The figure shows three views and two pictorial views of one solid part (mm, origin at its lowest corner). Answer the questions. A direction names the side the tool comes from. Coordinates: 2 decimals unless noted, no trailing zeros. Loops run counter-clockwise (first coordinate to the right, second up) from the corner with the lowest first, then second, coordinate; pieces in that order, holes last. Notation, with made-up numbers: (1, 1.25) - (12, 1.25) arc R34 ccw to (12, 32.25) - close; hole circle Ø5 at (-6, 56.25). An arc over 180 degrees is marked (long way). Return JSON: item names as keys, results as strings. Group by question number.
1. Section C-C (y = 31.5) is taken. Write down the section's boundary in (x, z), and give its area (3 significant figures).
2. The mould has two halves that part along X. Classify the marked faces 3 and 4: pulls with the +X half, pulls with the -X half, needs draft (parallel to the pull), parting line crosses it, or undercut.
3. Which of the six approach directions +Z, -Z, +X, -X, +Y, -Y give full straight-line access (tool end or side, diameter ignored) to the marked faces 1 and 2?
4. Section A-A (z = 31.75) is taken. Write down the section's boundary in (x, y) (3 decimals).
5. Find the intervals of material crossed by line 1 along Y through (x, z) = (59, 41) (3 decimals); line 2 along Y through (x, z) = (10, 31); line 3 along X through (y, z) = (13.5, 36), in increasing order.
6. Each of these flat-tipped pins is pushed along its axis until it touches: P1, Ø6, axis at y = 27.5, z = 26.5, coming from the -X side; P2, Ø1, axis at x = 52, z = 36.5, coming from the +Y side; P3, Ø6, axis at y = 22.5, z = 36.5, coming from the -X side. Where does it stop, or does it pass through?
7. Section B-B (x = 31.75) is taken. Write down the section's boundary in (y, z) (3 decimals), and give its area (3 significant figures).
8. Section D-D (x = 59.5) is taken. Write down the section's boundary in (y, z) (3 decimals).
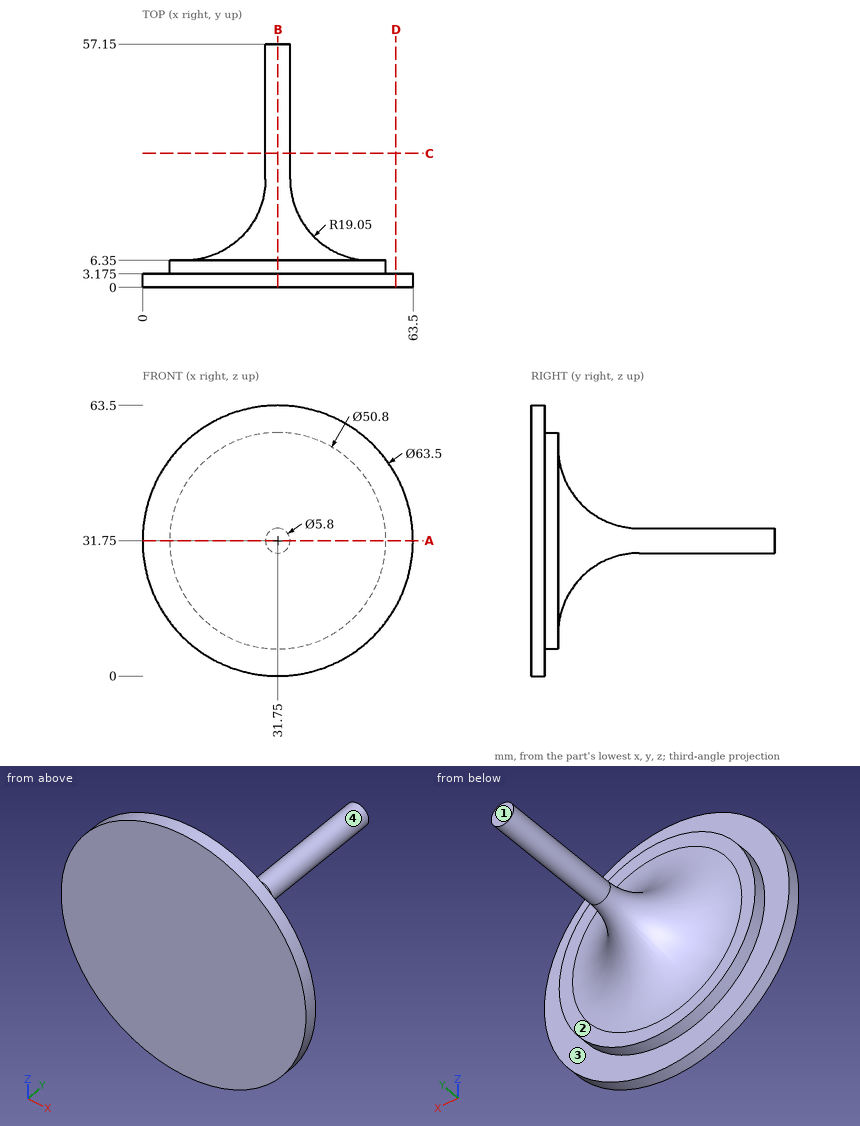
The answers:
{
 "1": {"outline": "circle Ø5.8 at (31.75, 31.75)", "area": "26.4 mm2"},
 "2": {"face 3": "needs draft", "face 4": "parting line crosses it"},
 "3": {"face 1": "+Z, -Z, +X, -X, +Y", "face 2": "+Y"},
 "4": {"outline": "(0, 0) - (63.5, 0) - (63.5, 3.175) - (57.15, 3.175) - (57.15, 6.35) - (53.7, 6.35) arc R19.05 cw to (34.65, 25.4) - (34.65, 57.15) - (28.85, 57.15) - (28.85, 25.4) arc R19.05 cw to (9.8, 6.35) - (6.35, 6.35) - (6.35, 3.175) - (0, 3.175) - close"},
 "5": {"line 1": "y = 0 to 3.175", "line 2": "y = 0 to 6.35", "line 3": "x = 26.09 to 37.41"},
 "6": {"P1": "stops at x = 29.92", "P2": "stops at y = 6.42", "P3": "stops at x = 29.06"},
 "7": {"outline": "(0, 0) - (3.175, 0) - (3.175, 6.35) - (6.35, 6.35) - (6.35, 9.8) arc R19.05 cw to (25.4, 28.85) - (57.15, 28.85) - (57.15, 34.65) - (25.4, 34.65) arc R19.05 cw to (6.35, 53.7) - (6.35, 57.15) - (3.175, 57.15) - (3.175, 63.5) - (0, 63.5) - close", "area": "813 mm2"},
 "8": {"outline": "(0, 16.323) - (3.175, 16.323) - (3.175, 47.177) - (0, 47.177) - close"}
}
